The drawing under review shows one solid part. Ordinate dimensions are in mm from its lowest x, y, z. Round coordinates to 2 decimals unless told otherwise and drop trailing zeros. Write each loop counter-clockwise with the first axis right and the second up, starting at its lowest first coordinate (ties: lowest second). Pieces come first, ordered by that corner, then holes. Notation, with made-up numbers: (70, -24.75) -> (114, -24.75) arc R38 cw to (114, 14.25) -> close; hole circle Ø2 at (63.25, 15.25). An arc over 180 degrees is marked (long way). Write item = value, one per line. Start each with the question number.
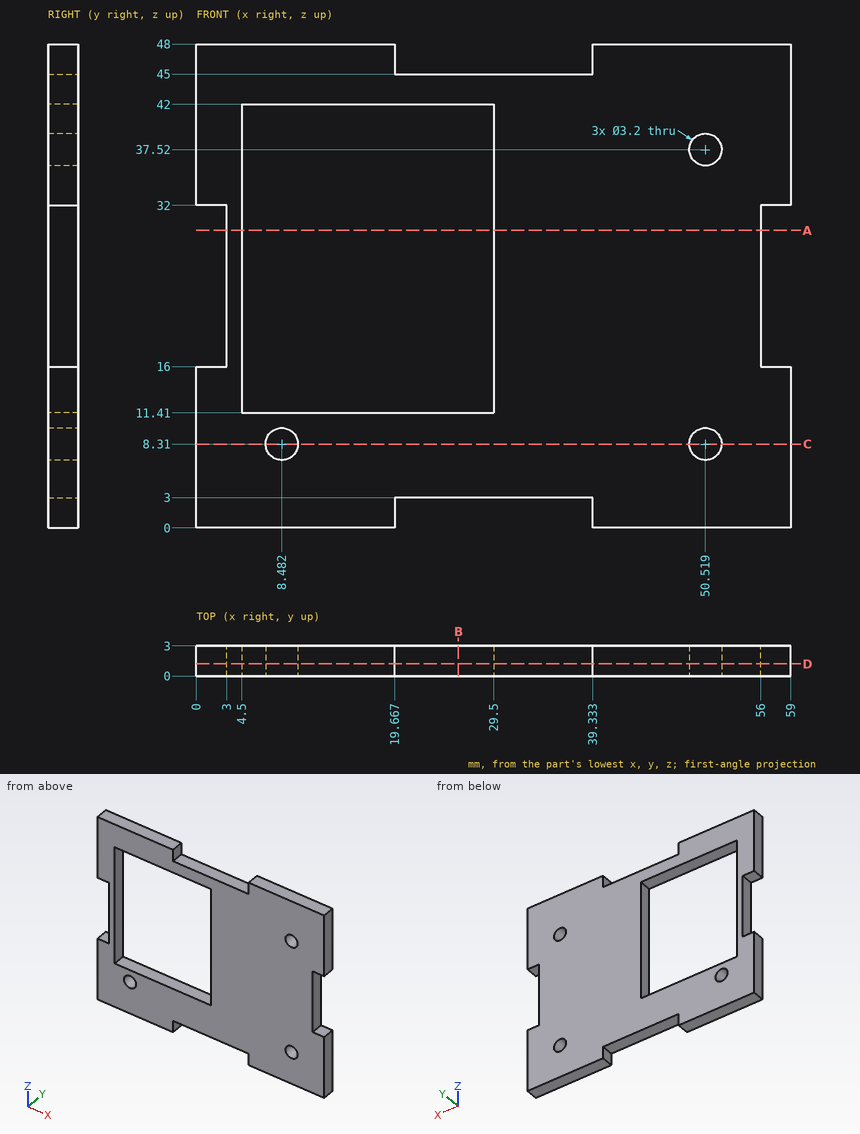
1. Wall thickness on L1, parallel to X at y = 0.7, z = 8.31; L2, parallel to X at y = 2.35, z = 37.52; L3, parallel to Z at x = 15, y = 2.7: over which ranges is each line inside the solid? List them lowest first. Write a range as from..to.
2. Consider section D-D, the plane y = 1.2. Give the boundary of the cut face in (x, z).
3. Consider section A-A, the plane z = 29.5. Give the boundary of the cut face in (x, y).
4. Clearance check with flat-ended pins moving along their axes: pin 1 Ø1 at (y, z) = (2, 35) entering from -X; pin 2 Ø0.9 at (x, y) = (29, 2) entering from +Z; pin 3 Ø1.9 at (x, z) = (50.52, 37.52) entering from -Y; pin 4 Ø1.5 at (y, z) = (1, 20.5) entering from -X. State where each tip first meets the part, or that it passes through.
5. Consider section C-C, the plane z = 8.31. Give the boundary of the cut face in (x, y), then the cut area to 3 significant figures.
6. Consider section B-B, the plane x = 26. Give the boundary of the cut face in (y, z).
Outcome:
q1.L1 = 0..6.88, 10.08..48.92, 52.12..59
q1.L2 = 0..4.5, 29.5..48.92, 52.12..59
q1.L3 = 0..11.41, 42..48
q2.outline = (0, 0) -> (19.67, 0) -> (19.67, 3) -> (39.33, 3) -> (39.33, 0) -> (59, 0) -> (59, 16) -> (56, 16) -> (56, 32) -> (59, 32) -> (59, 48) -> (39.33, 48) -> (39.33, 45) -> (19.67, 45) -> (19.67, 48) -> (0, 48) -> (0, 32) -> (3, 32) -> (3, 16) -> (0, 16) -> close; hole (4.5, 11.41) -> (29.5, 11.41) -> (29.5, 42) -> (4.5, 42) -> close; hole circle Ø3.2 at (8.48, 8.31); hole circle Ø3.2 at (50.52, 8.31); hole circle Ø3.2 at (50.52, 37.52)
q3.outline = (3, 0) -> (4.5, 0) -> (4.5, 3) -> (3, 3) -> close; (29.5, 0) -> (56, 0) -> (56, 3) -> (29.5, 3) -> close
q4.pin_1 = 0
q4.pin_2 = 45
q4.pin_3 = through
q4.pin_4 = 3
q5.outline = (0, 0) -> (6.88, 0) -> (6.88, 3) -> (0, 3) -> close; (10.08, 0) -> (48.92, 0) -> (48.92, 3) -> (10.08, 3) -> close; (52.12, 0) -> (59, 0) -> (59, 3) -> (52.12, 3) -> close
q5.area = 158 mm2
q6.outline = (0, 3) -> (3, 3) -> (3, 11.41) -> (0, 11.41) -> close; (0, 42) -> (3, 42) -> (3, 45) -> (0, 45) -> close
